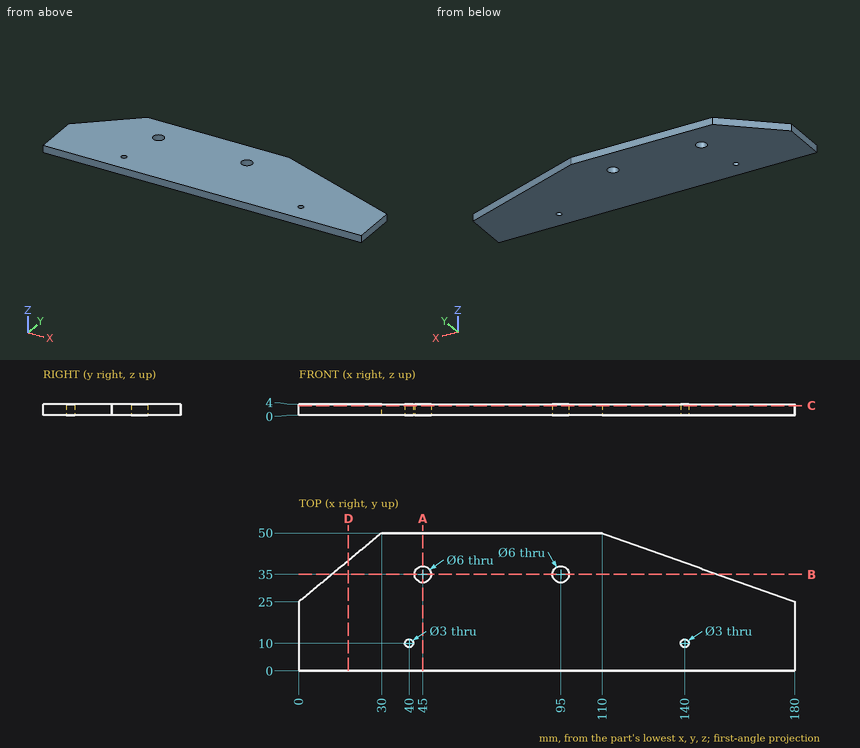
Study the drawing (mm; zero at the part's minimum x, y, z) and answer. Give positions to 0.01 mm unless a question says otherwise; leave off trailing zeros. Loops run counter-clockwise (first coordinate to the right, second up) from the corner with the lowest first, then second, coordinate; pieces in that order, holes last. Notation, with made-up numbers: (68, 15) -> (116, 15) arc R24 ccw to (116, 41) -> close; hole circle Ø1 at (-4.5, 65). An arc over 180 degrees is marked (long way). Use a Markdown table: item, result. Add a question column.
1) Each of these flat-tipped pins is pushed along its axis until it touches: P1, Ø8, axis at x = 73, y = 14, coming from the -Z side; P2, Ø12, axis at x = 157.5, y = 42.5, coming from the +Z side; P3, Ø2, axis at x = 124.5, z = 2.5, coming from the +Y side. Where does it stop, or does it pass through?
2) Consider line 1 along Y through (x, z) = (45, 1.7); line 2 along X through (y, z) = (11, 3.7); line 3 along Y through (x, z) = (140, 2). Determine where each line is inside the solid, lowest interval first.
3) The part is cut by section C-C, the plane z = 3.4. Determine the outline of the cut face in (x, y).
4) The part is cut by section D-D, the plane x = 18. Determine the outline of the cut face in (y, z).
5) The part is cut by section B-B, the plane y = 35. Determine the outline of the cut face in (x, z), plus the area to 3 significant figures.
6) The part is cut by section A-A, the plane x = 45. Determine the outline of the cut face in (y, z).
Reported:
| question | item | result |
|---|---|---|
| 1 | P1 | stops at z = 0 |
| 1 | P2 | passes through |
| 1 | P3 | stops at y = 45.18 |
| 2 | line 1 | y = 0 to 32, 38 to 50 |
| 2 | line 2 | x = 0 to 38.88, 41.12 to 138.88, 141.12 to 180 |
| 2 | line 3 | y = 0 to 8.5, 11.5 to 39.29 |
| 3 | outline | (0, 0) -> (180, 0) -> (180, 25) -> (110, 50) -> (30, 50) -> (0, 25) -> close; hole circle Ø3 at (40, 10); hole circle Ø6 at (45, 35); hole circle Ø6 at (95, 35); hole circle Ø3 at (140, 10) |
| 4 | outline | (0, 0) -> (40, 0) -> (40, 4) -> (0, 4) -> close |
| 5 | outline | (12, 0) -> (42, 0) -> (42, 4) -> (12, 4) -> close; (48, 0) -> (92, 0) -> (92, 4) -> (48, 4) -> close; (98, 0) -> (152, 0) -> (152, 4) -> (98, 4) -> close |
| 5 | area | 512 mm^2 |
| 6 | outline | (0, 0) -> (32, 0) -> (32, 4) -> (0, 4) -> close; (38, 0) -> (50, 0) -> (50, 4) -> (38, 4) -> close |
